from build123d import *

# Parameters (mm, degrees)
SKETCH1_W                = 38.1
SKETCH1_H                = 63.5
BOSS_EXTRUDE1_DEPTH      = 3.175
F_8_CLEARANCE_HOLE1_D    = 4.4958
F_5_16_CLEARANCE_HOLE1_D = 8.2042
SKETCH6_W                = 40.64
SKETCH6_H                = 66.04
CUT_EXTRUDE1_DEPTH       = 3.175


with BuildPart() as part:
    # Sketch1 → Boss-Extrude1 (new body)
    with BuildSketch(Plane(origin=(0, 0, 0), x_dir=(1, 0, 0), z_dir=(0, 1, 0))):
        with Locations((19.05, 31.75)):
            Rectangle(SKETCH1_W, SKETCH1_H)
    extrude(amount=BOSS_EXTRUDE1_DEPTH)

    # #8 Clearance Hole1 (through all)
    with Locations(Plane(origin=(0, 3.175, 0), x_dir=(1, 0, 0), z_dir=(0, 1, 0))):
        with Locations((19.05, 31.75)):
            Hole(F_8_CLEARANCE_HOLE1_D / 2)

    # 5/16 Clearance Hole1 (through all)
    with Locations(Plane(origin=(0, 3.175, 0), x_dir=(1, 0, 0), z_dir=(0, 1, 0))):
        with Locations((19.05, 9.525), (19.05, 53.975)):
            Hole(F_5_16_CLEARANCE_HOLE1_D / 2)

    # Sketch6 → Cut-Extrude1 (cut)
    with BuildSketch(Plane(origin=(0, 3.175, 0), x_dir=(1, 0, 0), z_dir=(0, 1, 0))):
        with Locations((19.05, 31.75)):
            Rectangle(SKETCH6_W, SKETCH6_H)
        with BuildLine():
            Line((27.655912775, 58.057142857), (36.26182555, 39.914285714))
            ThreePointArc((36.26182555, 39.914285714), (38.1, 31.75), (36.26182555, 23.585714286))
            Line((36.26182555, 23.585714286), (27.655912775, 5.442857143))
            ThreePointArc((27.655912775, 5.442857143), (19.05, 0), (10.444087225, 5.442857143))
            Line((10.444087225, 5.442857143), (1.83817445, 23.585714286))
            ThreePointArc((1.83817445, 23.585714286), (0, 31.75), (1.83817445, 39.914285714))
            Line((1.83817445, 39.914285714), (10.444087225, 58.057142857))
            ThreePointArc((10.444087225, 58.057142857), (19.05, 63.5), (27.655912775, 58.057142857))
        make_face(mode=Mode.SUBTRACT)
    extrude(amount=-CUT_EXTRUDE1_DEPTH, mode=Mode.SUBTRACT)


solid = part.part
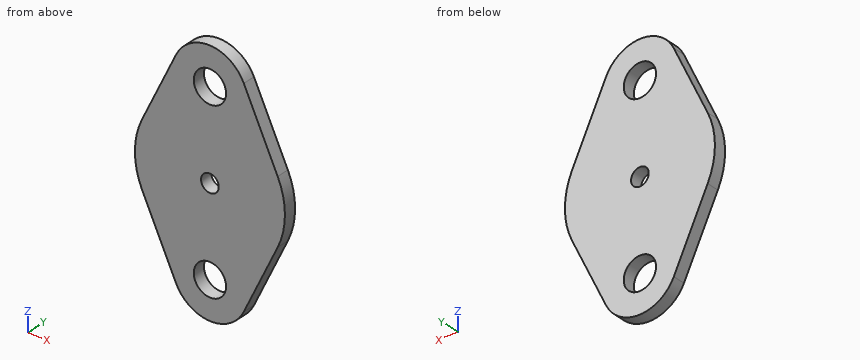
Design review of the part built by this model. Coordinates are the model's own, in mm. Round coordinates to 2 decimals unless told otherwise and drop trailing zeros. Loops run counter-clockwise (first coordinate to the right, second up) from the corner with the lowest first, then second, coordinate; pieces in that order, holes last. Notation, with made-up numbers: (-25, 15.25) - (-7, 15.25) arc R21 ccw to (-7, 48.25) - close; hole circle Ø2 at (-11.5, 10). An arc over 180 degrees is marked (long way). One line per item, written item: value. Start each with the question number.
1) Consider section C-C on y = 1.8. Give the boundary of the cut face in (x, z) (3 decimals).
2) To check wall thickness, follow L1, parallel to Z at x = 19.05, y = 0.7; L2, parallel to X at y = 1.9, z = -31.75; L3, parallel to Z at x = 17, y = 1.6. State the ranges of each line that lie inside material, in increasing order. Write a range as from..to.
3) Consider section B-B on x = 19.05. Give the boundary of the cut face in (y, z) (3 decimals).
4) Consider section D-D on z = -57. Give the boundary of the cut face in (x, y) (3 decimals).
5) Consider section A-A on z = -31.75. Give the boundary of the cut face in (x, y) (3 decimals), then the cut area to 3 significant figures.
6) Insertion check: pin 1 Ø7 at (x, z) = (19.05, -31.75) entering from +Y (3 decimals); pin 2 Ø1.5 at (x, y) = (31, 0.5) entering from -Z; pin 3 Ø5 at (x, z) = (19.05, -53.975) entering from -Y (3 decimals). Each pin has a flat end and moves straight along its axis. Give the tip position at first contact, or say it passes through.
Reported:
1. outline: (1.838, -39.914) - (10.444, -58.057) arc R9.525 ccw to (27.656, -58.057) - (36.262, -39.914) arc R19.05 ccw to (36.262, -23.586) - (27.656, -5.443) arc R9.525 ccw to (10.444, -5.443) - (1.838, -23.586) arc R19.05 ccw to start; hole circle Ø8.204 at (19.05, -53.975); hole circle Ø8.204 at (19.05, -9.525); hole circle Ø4.496 at (19.05, -31.75)
2. L1: z = -63.5..-58.08, -49.87..-34, -29.5..-13.63, -5.42..0
2. L2: x = 0..16.8, 21.3..38.1
2. L3: z = -63.28..-57.53, -50.42..-32.67, -30.83..-13.08, -5.97..-0.22
3. outline: (0, -63.5) - (3.175, -63.5) - (3.175, -58.077) - (0, -58.077) - close; (0, -49.873) - (3.175, -49.873) - (3.175, -33.998) - (0, -33.998) - close; (0, -29.502) - (3.175, -29.502) - (3.175, -13.627) - (0, -13.627) - close; (0, -5.423) - (3.175, -5.423) - (3.175, 0) - (0, 0) - close
4. outline: (9.943, 0) - (16.279, 0) - (16.279, 3.175) - (9.943, 3.175) - close; (21.821, 0) - (28.157, 0) - (28.157, 3.175) - (21.821, 3.175) - close
5. outline: (0, 0) - (16.802, 0) - (16.802, 3.175) - (0, 3.175) - close; (21.298, 0) - (38.1, 0) - (38.1, 3.175) - (21.298, 3.175) - close
5. area: 107 mm^2
6. pin 1: stops at y = 3.175
6. pin 2: stops at z = -52.59
6. pin 3: passes through
